```python
from build123d import *

# Parameters (mm, degrees)
SKETCH1_W              = 10
SKETCH1_H              = 5
CHAMFER1_SIZE          = 0.2
M4_TAPPED_HOLE1_REACH  = 22.736
M4_TAPPED_HOLE1_BORE_R = 1.65


with BuildPart() as part:
    # Sketch1 → Revolve1 (revolve)
    with BuildSketch(Plane.XY, mode=Mode.PRIVATE) as revolve1_sk:
        with Locations((0, 6.5)):
            Rectangle(SKETCH1_W, SKETCH1_H)
    revolve(revolve1_sk.sketch.rotate(Axis((0, 0, 0), (-1, 0, 0)), 90), axis=Axis((0, 0, 0), (-1, 0, 0)))

    # Chamfer1
    chamfer1_edges = [part.edges().sort_by_distance(p)[0] for p in [
        (5, 0, 9),
        (-5, 0, 9),
    ]]
    chamfer(chamfer1_edges, length=CHAMFER1_SIZE)

    # M4 Tapped Hole1 bore → M4 Tapped Hole1 (cut, up to next)
    with BuildSketch(Plane(origin=(0, 9, 0), x_dir=(1, 0, 0), z_dir=(0, 1, 0)), mode=Mode.PRIVATE) as m4_tapped_hole1_sk1:
        Circle(M4_TAPPED_HOLE1_BORE_R)
    m4_tapped_hole1_tool1 = extrude(m4_tapped_hole1_sk1.sketch, amount=-M4_TAPPED_HOLE1_REACH, mode=Mode.PRIVATE) & part.part
    add(m4_tapped_hole1_tool1.solids().sort_by_distance((0, 9, 0))[0], mode=Mode.SUBTRACT)


solid = part.part
```
Part model, mm, in its own coordinate system. Coordinates: 2 decimals unless noted, no trailing zeros. Write each loop counter-clockwise with the first axis right and the second up, starting at its lowest first coordinate (ties: lowest second). Pieces come first, ordered by that corner, then holes.
Item 1: Slice it at B-B (y = 0). Write the cut outline in (x, z).
Item 2: Pin check, flat tips, straight feed: pin 1 (2 mm diameter, centred on y = -6, z = 6.5, fed in from +X); pin 2 (4 mm diameter, centred on x = 1.5, y = 4.5, fed in from -Z). Stop position of each tip, or through.
Item 3: Slice it at A-A (z = 0). Write the cut outline in (x, y), and give its area (3 significant figures).
Item 4: Mould opens along Z. For faces 1 (the face through (0.07, -3.373, -2.15)), 2 (the face through (-5, 2, 4)), 3 (the face through (1.524, 6.36, 0.632)), 4 (the face through (0.067, -6.083, 6.633)) say: released by +Z, released by -Z, zero draft, split by the parting line, or undercut.
Item 5: Slice it at C-C (x = 3). Write the cut outline in (y, z), and give its area (3 significant figures).
Item 6: Slice it at D-D (x = 0). Write the cut outline in (y, z).
Item 7: Probe line 1 (Y direction, x = 3, z = 0); line 2 (X direction, y = 7.1, z = 0); line 3 (Z direction, x = -3.75, y = 2.25). List the from-to ranges inside material, lowest first.
Results found:
1. outline: (-5, -8.8) - (-4.8, -9) - (4.8, -9) - (5, -8.8) - (5, -4) - (-5, -4) - close; (-5, 4) - (5, 4) - (5, 8.8) - (4.8, 9) - (-4.8, 9) - (-5, 8.8) - close
2. pin 1: stops at x = 5
2. pin 2: stops at z = -8.65
3. outline: (-5, -8.8) - (-4.8, -9) - (4.8, -9) - (5, -8.8) - (5, -4) - (-5, -4) - close; (-5, 4) - (-1.65, 4) - (-1.65, 9) - (-4.8, 9) - (-5, 8.8) - close; (1.65, 4) - (5, 4) - (5, 8.8) - (4.8, 9) - (1.65, 9) - close
3. area: 83.4 mm2
4. face 1: undercut
4. face 2: zero draft
4. face 3: undercut
4. face 4: split by the parting line
5. outline: circle Ø18 at (0, 0); hole circle Ø8 at (0, 0)
5. area: 204 mm2
6. outline: (3.64, -1.65) arc R4 cw (long way) to (3.64, 1.65) - (8.85, 1.65) arc R9 ccw (long way) to (8.85, -1.65) - close
7. line 1: y = -9 to -4, 4 to 9
7. line 2: x = -5 to -1.65, 1.65 to 5
7. line 3: z = -8.71 to -3.31, 3.31 to 8.71
